Geometry: final body of the model. Coordinates: model frame, mm. Face numbers are marked on the shaded views. Coordinates: 2 decimals unless noted, no trailing zeros. Loops run counter-clockwise (first coordinate to the right, second up) from the corner with the lowest first, then second, coordinate; pieces in that order, holes last. Notation, with made-up numbers: (-34.75, 75.5) - (-25.75, 75.5) arc R15 ccw to (-25.75, 90.5) - close; hole circle Ø5 at (75, 69). An arc over 180 degrees is marked (long way). Put each result on its own line as item: value. Start each with the question number.
1) Contact query for a flat-ended pin moving along its axis: pin 1 Ø3 at (x, z) = (72, -80) entering from +Y. Output: stop coordinate, or through.
2) Material intervals for line 1 along Y through (x, z) = (28, -99.5); line 2 along X through (y, z) = (11.9, -108.6); line 3 along Z through (x, y) = (14.5, 4.25), sorted ascending. Write a range as from..to.
3) Draft query along Z for the marked faces 1 and 2. Return one class per face: +Z half, -Z half, draft (parallel to the pull), parting line (faces both ways), or undercut.
4) Section D-D on z = -57. Output: boundary loops of the cut face in (x, y) (3 decimals), and give its area (3 significant figures).
5) Section C-C on z = -8.5. Output: boundary loops of the cut face in (x, y).
6) Section A-A on z = -78. Output: boundary loops of the cut face in (x, y) (3 decimals).
7) Section B-B on x = 40.5. Output: boundary loops of the cut face in (y, z) (3 decimals).
```python
from build123d import *

# Parameters (mm, degrees)
SKETCH1_W           = 126
SKETCH1_H           = 126
BOSS_EXTRUDE1_DEPTH = 5
SKETCH3_R           = 12.5
BOSS_EXTRUDE2_DEPTH = 7.5
SKETCH4_R           = 3.45
CUT_EXTRUDE1_DEPTH  = 11.5
SKETCH6_R           = 3
CUT_EXTRUDE2_DEPTH  = 179.628805068
CHAMFER1_SIZE       = 10
CHAMFER1_SIZE_2     = 7.26542528
SKETCH7_R           = 2.75
SKETCH7_R_2         = 2.625
SKETCH7_R_3         = 2.375
CUT_EXTRUDE3_DEPTH  = 179.348675353
CUT_EXTRUDE4_DEPTH  = 179.348675353


with BuildPart() as part:
    # Sketch1 → Boss-Extrude1 (new body)
    with BuildSketch(Plane(origin=(0, 0, 0), x_dir=(1, 0, 0), z_dir=(0, 1, 0))):
        with Locations((63, 63)):
            Rectangle(SKETCH1_W, SKETCH1_H)
    extrude(amount=BOSS_EXTRUDE1_DEPTH)

    # Sketch3 → Boss-Extrude2 (add)
    with BuildSketch(Plane(origin=(0, 5, 0), x_dir=(1, 0, 0), z_dir=(0, 1, 0))):
        with Locations(Location((108.6, 108.6, 0), (0, 0, 90))):
            Circle(SKETCH3_R)
    extrude(amount=BOSS_EXTRUDE2_DEPTH)

    # Sketch4 → Cut-Extrude1 (cut)
    with BuildSketch(Plane.XZ):
        with Locations(Location((108.6, -108.6, 0), (0, 0, 270))):
            Circle(SKETCH4_R)
    extrude(amount=-CUT_EXTRUDE1_DEPTH, mode=Mode.SUBTRACT)

    # Sketch6 → Cut-Extrude2 (cut, through all)
    with BuildSketch(Plane(origin=(0, 12.5, 0), x_dir=(1, 0, 0), z_dir=(0, 1, 0))):
        with Locations(Location((108.6, 108.6, 0), (0, 0, 270))):
            Circle(SKETCH6_R)
    extrude(amount=-CUT_EXTRUDE2_DEPTH, mode=Mode.SUBTRACT)

    # Chamfer1
    # the kernel refuses this chamfer: 10, 7.26542528 mm, written as the material it takes off along each edge
    with BuildSketch(Plane(origin=(108.6, 12.5, -108.6), x_dir=(0, 0, -1), z_dir=(1, 0, 0))) as chamfer1_piece_1_section:
        Polygon((12.5, -CHAMFER1_SIZE), (12.5 - CHAMFER1_SIZE_2, 0), (12.5, 0), align=None)
    chamfer1_piece_1 = revolve(axis=Axis((108.6, 12.5, -108.6), (0, 1, 0)), mode=Mode.PRIVATE)
    chamfer1_piece_1 = split(chamfer1_piece_1, bisect_by=Plane(origin=(108.6, 5, -100.650989912), z_dir=(0, 1, 0)), keep=Keep.TOP, mode=Mode.PRIVATE)
    add(chamfer1_piece_1, mode=Mode.SUBTRACT)

    # Sketch7 → Cut-Extrude3 (cut, through all)
    with BuildSketch(Plane(origin=(0, 5, 0), x_dir=(1, 0, 0), z_dir=(0, 1, 0))):
        with Locations(Location((55.375, 63, 0), (0, 0, 270))):
            Circle(SKETCH7_R)
        with Locations(Location((70.5, 63, 0), (0, 0, 270))):
            Circle(SKETCH7_R_2)
        with Locations(Location((40.5, 63, 0), (0, 0, 270))):
            Circle(SKETCH7_R_3)
        with Locations(Location((85.5, 63, 0), (0, 0, 270))):
            Circle(SKETCH7_R_2)
        with Locations(Location((25.625, 63, 0), (0, 0, 270))):
            Circle(SKETCH7_R)
        with Locations(Location((100.625, 63, 0), (0, 0, 270))):
            Circle(SKETCH7_R)
        with Locations(Location((25.625, 48, 0), (0, 0, 270))):
            Circle(SKETCH7_R)
        with Locations(Location((40.5, 48, 0), (0, 0, 270))):
            Circle(SKETCH7_R_3)
        with Locations(Location((55.375, 48, 0), (0, 0, 270))):
            Circle(SKETCH7_R)
        with Locations(Location((70.5, 48, 0), (0, 0, 270))):
            Circle(SKETCH7_R_2)
        with Locations(Location((85.5, 48, 0), (0, 0, 270))):
            Circle(SKETCH7_R_2)
        with Locations(Location((100.625, 48, 0), (0, 0, 270))):
            Circle(SKETCH7_R)
        with Locations(Location((25.625, 33, 0), (0, 0, 270))):
            Circle(SKETCH7_R)
        with Locations(Location((40.5, 33, 0), (0, 0, 270))):
            Circle(SKETCH7_R_3)
        with Locations(Location((55.375, 33, 0), (0, 0, 270))):
            Circle(SKETCH7_R)
        with Locations(Location((70.5, 33, 0), (0, 0, 270))):
            Circle(SKETCH7_R_2)
        with Locations(Location((85.5, 33, 0), (0, 0, 270))):
            Circle(SKETCH7_R_2)
        with Locations(Location((100.625, 33, 0), (0, 0, 270))):
            Circle(SKETCH7_R)
        with Locations(Location((25.625, 18, 0), (0, 0, 270))):
            Circle(SKETCH7_R)
        with Locations(Location((40.5, 18, 0), (0, 0, 270))):
            Circle(SKETCH7_R_3)
        with Locations(Location((55.375, 18, 0), (0, 0, 270))):
            Circle(SKETCH7_R)
        with Locations(Location((70.5, 18, 0), (0, 0, 270))):
            Circle(SKETCH7_R_2)
        with Locations(Location((85.5, 18, 0), (0, 0, 270))):
            Circle(SKETCH7_R_2)
        with Locations(Location((100.625, 18, 0), (0, 0, 270))):
            Circle(SKETCH7_R)
        with Locations(Location((25.625, 78, 0), (0, 0, 270))):
            Circle(SKETCH7_R)
        with Locations(Location((40.5, 78, 0), (0, 0, 270))):
            Circle(SKETCH7_R_3)
        with Locations(Location((55.375, 78, 0), (0, 0, 270))):
            Circle(SKETCH7_R)
        with Locations(Location((70.5, 78, 0), (0, 0, 270))):
            Circle(SKETCH7_R_2)
        with Locations(Location((85.5, 78, 0), (0, 0, 270))):
            Circle(SKETCH7_R_2)
        with Locations(Location((100.625, 78, 0), (0, 0, 270))):
            Circle(SKETCH7_R)
        with Locations(Location((25.625, 93, 0), (0, 0, 270))):
            Circle(SKETCH7_R)
        with Locations(Location((40.5, 93, 0), (0, 0, 270))):
            Circle(SKETCH7_R_3)
        with Locations(Location((55.375, 93, 0), (0, 0, 270))):
            Circle(SKETCH7_R)
        with Locations(Location((70.5, 93, 0), (0, 0, 270))):
            Circle(SKETCH7_R_2)
        with Locations(Location((85.5, 93, 0), (0, 0, 270))):
            Circle(SKETCH7_R_2)
        with Locations(Location((100.625, 93, 0), (0, 0, 270))):
            Circle(SKETCH7_R)
    extrude(amount=-CUT_EXTRUDE3_DEPTH, mode=Mode.SUBTRACT)

    # Sketch8 → Cut-Extrude4 (cut, through all)
    with BuildSketch(Plane(origin=(0, 5, 0), x_dir=(1, 0, 0), z_dir=(0, 1, 0))):
        Polygon((70.5, 100.747162737), (63, 108.375), (55.49988754, 100.747162737), align=None)
        Polygon((108.375, 63), (115.875, 55.5), (108.375, 48), align=None)
        Polygon((55.5, 10.375), (63, 2.75), (70.5, 10.375), align=None)
        Polygon((17.875, 63), (17.875, 48), (10.125, 55.5), align=None)
    extrude(amount=-CUT_EXTRUDE4_DEPTH, mode=Mode.SUBTRACT)


solid = part.part
```
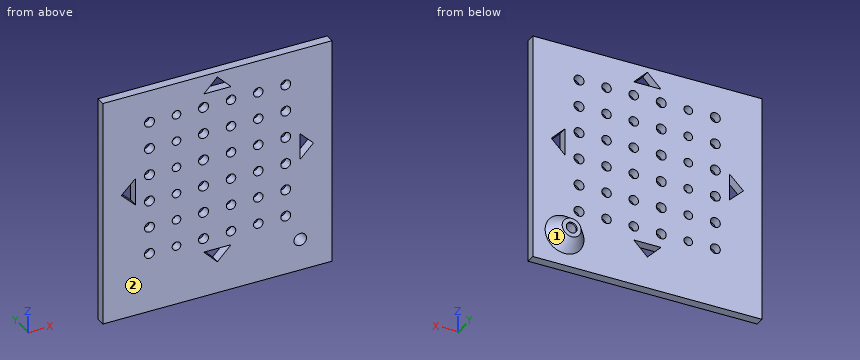
Answer block:
1. pin 1: stops at y = 5
2. line 1: y = 0..5
2. line 2: x = 102.93..105.6, 111.6..114.27
2. line 3: z = -126..-59.73, -51.27..0
3. face 1: parting line
3. face 2: draft
4. outline: (0, 0) - (11.675, 0) - (11.675, 5) - (0, 5) - close; (17.875, 0) - (108.375, 0) - (108.375, 5) - (17.875, 5) - close; (114.375, 0) - (126, 0) - (126, 5) - (114.375, 5) - close
4. area: 569 mm²
5. outline: (0, 0) - (57.34, 0) - (57.34, 5) - (0, 5) - close; (68.66, 0) - (126, 0) - (126, 5) - (68.66, 5) - close
6. outline: (0, 0) - (22.875, 0) - (22.875, 5) - (0, 5) - close; (28.375, 0) - (38.125, 0) - (38.125, 5) - (28.375, 5) - close; (42.875, 0) - (52.625, 0) - (52.625, 5) - (42.875, 5) - close; (58.125, 0) - (67.875, 0) - (67.875, 5) - (58.125, 5) - close; (73.125, 0) - (82.875, 0) - (82.875, 5) - (73.125, 5) - close; (88.125, 0) - (97.875, 0) - (97.875, 5) - (88.125, 5) - close; (103.375, 0) - (126, 0) - (126, 5) - (103.375, 5) - close
7. outline: (0, -126) - (5, -126) - (5, -95.375) - (0, -95.375) - close; (0, -90.625) - (5, -90.625) - (5, -80.375) - (0, -80.375) - close; (0, -75.625) - (5, -75.625) - (5, -65.375) - (0, -65.375) - close; (0, -60.625) - (5, -60.625) - (5, -50.375) - (0, -50.375) - close; (0, -45.625) - (5, -45.625) - (5, -35.375) - (0, -35.375) - close; (0, -30.625) - (5, -30.625) - (5, -20.375) - (0, -20.375) - close; (0, -15.625) - (5, -15.625) - (5, 0) - (0, 0) - close
